Build history of the part. All positions in model axes, mm. A direction names the side the tool comes from. Round coordinates to 2 decimals unless told otherwise and drop trailing zeros. Loops run counter-clockwise (first coordinate to the right, second up) from the corner with the lowest first, then second, coordinate; pieces in that order, holes last.
from build123d import *

# Parameters (mm, degrees)
BOSS_EXTRUDE1_DEPTH = 3
SKETCH3_W           = 3.2
SKETCH3_H           = 10.2
SKETCH3_W_2         = 10.2
SKETCH3_H_2         = 3.2
SKETCH3_H_3         = 7.372217102
CUT_EXTRUDE1_DEPTH  = 4


with BuildPart() as part:
    # Sketch1 → Boss-Extrude1 (new body)
    with BuildSketch(Plane(origin=(0, 0, 0), x_dir=(1, 0, 0), z_dir=(0, 1, 0))):
        with BuildLine():
            Line((-55.172217102, 43.501443346), (-41.872217102, 43.501443346))
            ThreePointArc((-41.872217102, 43.501443346), (-38.336683196, 42.036977252), (-36.872217102, 38.501443346))
            Line((-36.872217102, 38.501443346), (-36.872217102, -48.542990858))
            ThreePointArc((-36.872217102, -48.542990858), (-35.407751008, -52.078524764), (-31.872217102, -53.542990858))
            Line((-31.872217102, -53.542990858), (31.872217102, -53.542990858))
            ThreePointArc((31.872217102, -53.542990858), (35.407751008, -52.078524764), (36.872217102, -48.542990858))
            Line((36.872217102, -48.542990858), (36.872217102, 38.501443346))
            ThreePointArc((36.872217102, 38.501443346), (38.336683196, 42.036977252), (41.872217102, 43.501443346))
            Line((41.872217102, 43.501443346), (55.172217102, 43.501443346))
            Line((55.172217102, 43.501443346), (55.172217102, -66.842990858))
            Line((55.172217102, -66.842990858), (-55.172217102, -66.842990858))
            Line((-55.172217102, -66.842990858), (-55.172217102, 43.501443346))
        make_face()
    extrude(amount=-BOSS_EXTRUDE1_DEPTH)

    # Sketch3 → Cut-Extrude1 (cut, through all)
    with BuildSketch(Plane(origin=(0, 0, 0), x_dir=(1, 0, 0), z_dir=(0, 1, 0))):
        with Locations((53.672217102, -41.670773756)):
            Rectangle(SKETCH3_W, SKETCH3_H)
        Polygon((52.072217102, -56.570773756), (55.272217102, -56.570773756), (55.272217102, -66.942990858), (44.9, -66.942990858), (44.9, -63.742990858), (52.072217102, -63.742990858), align=None)
        with Locations((30, -65.342990858)):
            Rectangle(SKETCH3_W_2, SKETCH3_H_2)
        with Locations((53.672217102, 18.329226244)):
            Rectangle(SKETCH3_W, SKETCH3_H)
        with Locations((53.672217102, -1.670773756)):
            Rectangle(SKETCH3_W, SKETCH3_H)
        with Locations((53.672217102, 36.915334795)):
            Rectangle(SKETCH3_W, SKETCH3_H_3)
        with Locations((10, -65.342990858)):
            Rectangle(SKETCH3_W_2, SKETCH3_H_2)
        with Locations((53.672217102, -21.670773756)):
            Rectangle(SKETCH3_W, SKETCH3_H)
        with Locations((-53.672217102, 36.915334795)):
            Rectangle(SKETCH3_W, SKETCH3_H_3)
        with Locations((-10, -65.342990858)):
            Rectangle(SKETCH3_W_2, SKETCH3_H_2)
        with Locations((-53.672217102, -1.670773756)):
            Rectangle(SKETCH3_W, SKETCH3_H)
        with Locations((-53.672217102, 18.329226244)):
            Rectangle(SKETCH3_W, SKETCH3_H)
        with Locations((-30, -65.342990858)):
            Rectangle(SKETCH3_W_2, SKETCH3_H_2)
        Polygon((-44.9, -66.942990858), (-55.272217102, -66.942990858), (-55.272217102, -56.570773756), (-52.072217102, -56.570773756), (-52.072217102, -63.742990858), (-44.9, -63.742990858), align=None)
        with Locations((-53.672217102, -41.670773756)):
            Rectangle(SKETCH3_W, SKETCH3_H)
        with Locations((-53.672217102, -21.670773756)):
            Rectangle(SKETCH3_W, SKETCH3_H)
    extrude(amount=-CUT_EXTRUDE1_DEPTH, mode=Mode.SUBTRACT)


solid = part.part
(1) Which spindle directions (+Z, -Z, +X, -X, +Y, -Y) get a long thin tool onto all of the face, cutting with end or side? Do faces 1 (the face through (-36.872, -1, 4)), 2 (the face through (48, -1, 63.743)), 3 (the face through (-54, -1, 6.771)). Say none if no direction does.
Responses:
face 1: -Z, +Y, -Y
face 2: +Z, +X, +Y, -Y
face 3: -X, +Y, -Y
(2) Slice it at C-C on z = 50. List the corners of the cut face in (x, y).
Responses:
outline: (-55.17, -3) - (-36.66, -3) - (-36.66, 0) - (-55.17, 0) - close; (36.66, -3) - (55.17, -3) - (55.17, 0) - (36.66, 0) - close
(3) Slice it at B-B on x = -7. List the corners of the cut face in (y, z), plus the area to 3 significant figures.
Responses:
outline: (-3, 53.54) - (0, 53.54) - (0, 63.74) - (-3, 63.74) - close
area: 30.6 mm2
(4) Pin check, flat tips, straight feed: P1, Ø1.5, axis at x = -53, y = -1, coming from the +Z side; P2, Ø1.5, axis at y = -1.5, z = 66, coming from the -X side; P3, Ø0.9, axis at x = 12, y = -1, coming from the +Z side. Stop position of each tip, or through.
Responses:
P1: stops at z = 56.57
P2: stops at x = -44.9
P3: stops at z = 63.74
(5) Pull direction X, two halves, no side cores. Call faces 4 (the face through (-38.4, -1.5, -42.1)), 5 (the face through (55.172, -1, -42)), 6 (the face through (-54, -1, 16.571)): +X half, -X half, draft (parallel to the pull), parting line (faces both ways), or undercut.
Responses:
face 4: undercut
face 5: +X half
face 6: draft
(6) Slice it at A-A on z = -5.5. List the corners of the cut face in (x, y), plus the area to 3 significant figures.
Responses:
outline: (-55.17, -3) - (-36.87, -3) - (-36.87, 0) - (-55.17, 0) - close; (36.87, -3) - (55.17, -3) - (55.17, 0) - (36.87, 0) - close
area: 110 mm2
(7) Probe line 1 (X direction, y = -2.6, z = 38); line 2 (X direction, y = -1.45, z = 36); line 3 (Z direction, x = 0.5, y = -2.6). List the from-to ranges inside material, lowest first.
Responses:
line 1: x = -52.07 to -36.87, 36.87 to 52.07
line 2: x = -55.17 to -36.87, 36.87 to 55.17
line 3: z = 53.54 to 66.84
